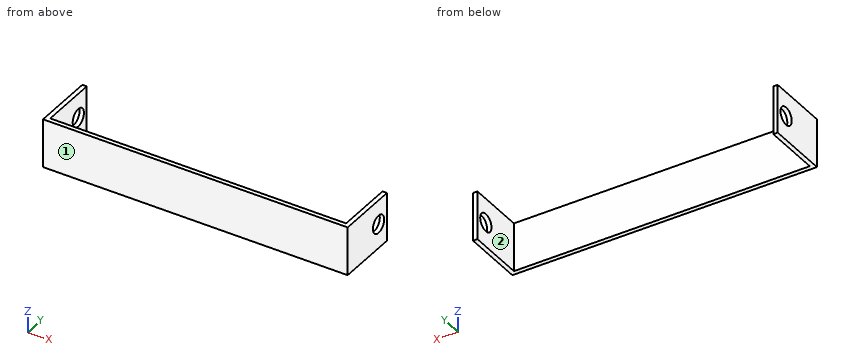
```python
from build123d import *

# Parameters (mm, degrees)
BOSS_EXTRUDE1_DEPTH      = 27.5
BOSS_EXTRUDE1_DEPTH_BACK = 27.5
SKETCH2_R                = 10
CUT_EXTRUDE1_DEPTH       = 346


with BuildPart() as part:
    # Sketch1 → Boss-Extrude1 (new body, two sides)
    with BuildSketch(Plane.XY) as boss_extrude1_sk:
        Polygon((-172.5, 0), (172.5, 0), (172.5, 70), (167.5, 70), (167.5, 5), (-167.5, 5), (-167.5, 70), (-172.5, 70), align=None)
    extrude(amount=BOSS_EXTRUDE1_DEPTH)
    extrude(boss_extrude1_sk.sketch, amount=-BOSS_EXTRUDE1_DEPTH_BACK)

    # Sketch2 → Cut-Extrude1 (cut, through all)
    with BuildSketch(Plane(origin=(172.5, 0, 0), x_dir=(0, 0, -1), z_dir=(1, 0, 0))):
        with Locations((0, 55)):
            Circle(SKETCH2_R)
    extrude(amount=-CUT_EXTRUDE1_DEPTH, mode=Mode.SUBTRACT)


solid = part.part
```
For this review, take the finished solid that the model builds, in its own axes (mm). Face numbers are marked on the shaded views. A direction names the side the tool comes from. Coordinates: 2 decimals unless noted, no trailing zeros. Write each loop counter-clockwise with the first axis right and the second up, starting at its lowest first coordinate (ties: lowest second). Pieces come first, ordered by that corner, then holes. Notation, with made-up numbers: (54, 30) -> (85, 30) arc R35 ccw to (85, 68) -> close; hole circle Ø11 at (80, 66.5). An arc over 180 degrees is marked (long way). Put each result on its own line as item: value.
Q1. Clearance check with a flat-ended pin moving along its axis: pin 1 Ø1.5 at (x, z) = (113.5, 2) entering from +Y. State where the tip first meets the part, or that it passes through.
From the geometry:
pin 1: stops at y = 5
Q2. Wall thickness on L1, parallel to X at y = 28, z = -5.5; L2, parallel to Y at x = 170, z = 0; L3, parallel to Y at x = 61, z = 17: over which ranges is each line inside the solid? List them lowest first.
From the geometry:
L1: x = -172.5 to -167.5, 167.5 to 172.5
L2: y = 0 to 45, 65 to 70
L3: y = 0 to 5
Q3. Tool access review of the marked faces 1 and 2: name each direction out of +Z, -Z, +X, -X, +Y, -Y from which nothing blocks a thin tool from reaching the whole face with its end or side.
From the geometry:
face 1: +Z, -Z, +X, -X, -Y
face 2: +Z, -Z, +Y
Q4. Take a section at D-D, the plane z = 16.5. State the section outline as (x, y) points, then the cut area to 4 significant figures.
From the geometry:
outline: (-172.5, 0) -> (172.5, 0) -> (172.5, 70) -> (167.5, 70) -> (167.5, 5) -> (-167.5, 5) -> (-167.5, 70) -> (-172.5, 70) -> close
area: 2,375 mm2
Q5. Take a section at A-A, the plane z = 0. State the section outline as (x, y) points, then the cut area to 4 significant figures.
From the geometry:
outline: (-172.5, 0) -> (172.5, 0) -> (172.5, 45) -> (167.5, 45) -> (167.5, 5) -> (-167.5, 5) -> (-167.5, 45) -> (-172.5, 45) -> close; (-172.5, 65) -> (-167.5, 65) -> (-167.5, 70) -> (-172.5, 70) -> close; (167.5, 65) -> (172.5, 65) -> (172.5, 70) -> (167.5, 70) -> close
area: 2,175 mm2
Q6. Take a section at B-B, the plane y = 55. State the section outline as (x, z) points.
From the geometry:
outline: (-172.5, -27.5) -> (-167.5, -27.5) -> (-167.5, -10) -> (-172.5, -10) -> close; (-172.5, 10) -> (-167.5, 10) -> (-167.5, 27.5) -> (-172.5, 27.5) -> close; (167.5, -27.5) -> (172.5, -27.5) -> (172.5, -10) -> (167.5, -10) -> close; (167.5, 10) -> (172.5, 10) -> (172.5, 27.5) -> (167.5, 27.5) -> close
Q7. Take a section at C-C, the plane y = 12.5. State the section outline as (x, z) points.
From the geometry:
outline: (-172.5, -27.5) -> (-167.5, -27.5) -> (-167.5, 27.5) -> (-172.5, 27.5) -> close; (167.5, -27.5) -> (172.5, -27.5) -> (172.5, 27.5) -> (167.5, 27.5) -> close
